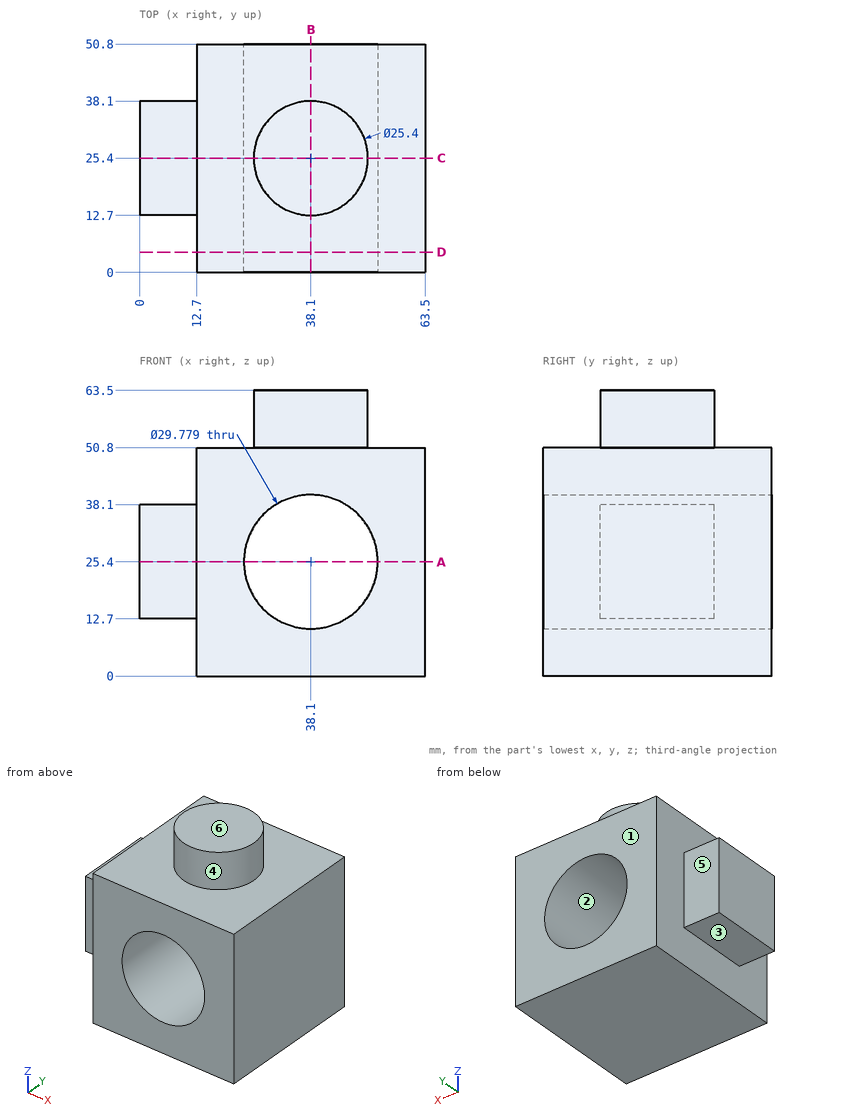
Drawing for the job (mm, zero at the part's lowest x, y, z). A direction names the side the tool comes from. Give positions to 0.01 mm unless a question says otherwise; leave off trailing zeros. Loops run counter-clockwise (first coordinate to the right, second up) from the corner with the lowest first, then second, coordinate; pieces in that order, holes last.
1) Probe line 1 along Z through (x, y) = (38.1, 15.5); line 2 along X through (y, z) = (23, 25); line 3 along Z through (x, y) = (38.1, 38.5). List the from-to ranges inside material, lowest first.
Values follow:
line 1: z = 0 to 10.51, 40.29 to 63.5
line 2: x = 0 to 23.22, 52.98 to 63.5
line 3: z = 0 to 10.51, 40.29 to 50.8
2) 3-axis set-ups, long thin cutter, end or side, ignore diameter. For the marked faces 4, 5 and 6: which of +Z, -Z, +X, -X, +Y, -Y reach the whole face in a straight line?
Values follow:
face 4: +Z
face 5: +Z, -Z, -X, +Y
face 6: +Z, +X, -X, +Y, -Y
3) Drop flat-ended pins along their axis: P1, Ø1.5, axis at x = 35.5, y = 13.5, coming from the -Z side; P2, Ø2, axis at y = 20.5, z = 52.5, coming from the +X side; P3, Ø1.5, axis at y = 42.5, z = 43.5, coming from the -X side; P4, Ø14, axis at x = 9, y = 29, coming from the +Z side. Give the stop position or say it passes through.
Values follow:
P1: stops at z = 0
P2: stops at x = 50.19
P3: stops at x = 12.7
P4: stops at z = 50.8
4) Two-plate mould, pull along Z, no slides. Class the marked faces 1, 2 and 3: released by +Z, released by -Z, zero draft, split by the parting line, or undercut.
Values follow:
face 1: zero draft
face 2: undercut
face 3: released by -Z
5) Band-saw the part on A-A on z = 25.4. List the corners of the cut face in (x, y).
Values follow:
outline: (0, 12.7) - (12.7, 12.7) - (12.7, 0) - (23.21, 0) - (23.21, 50.8) - (12.7, 50.8) - (12.7, 38.1) - (0, 38.1) - close; (52.99, 0) - (63.5, 0) - (63.5, 50.8) - (52.99, 50.8) - close
6) Band-saw the part on D-D on y = 4.5. List the corners of the cut face in (x, z), then the cut area to 3 significant figures.
Values follow:
outline: (12.7, 0) - (63.5, 0) - (63.5, 50.8) - (12.7, 50.8) - close; hole circle Ø29.78 at (38.1, 25.4)
area: 1,880 mm2
7) Band-saw the part on B-B on x = 38.1. List the corners of the cut face in (y, z).
Values follow:
outline: (0, 0) - (50.8, 0) - (50.8, 10.51) - (0, 10.51) - close; (0, 40.29) - (50.8, 40.29) - (50.8, 50.8) - (38.1, 50.8) - (38.1, 63.5) - (12.7, 63.5) - (12.7, 50.8) - (0, 50.8) - close
8) Band-saw the part on C-C on y = 25.4. List the corners of the cut face in (x, z), then the cut area to 3 significant figures.
Values follow:
outline: (0, 12.7) - (12.7, 12.7) - (12.7, 0) - (63.5, 0) - (63.5, 50.8) - (50.8, 50.8) - (50.8, 63.5) - (25.4, 63.5) - (25.4, 50.8) - (12.7, 50.8) - (12.7, 38.1) - (0, 38.1) - close; hole circle Ø29.78 at (38.1, 25.4)
area: 2,530 mm2
